Here's how the part is built. I have some questions about the finished solid (model axes, mm). Face numbers are marked on the shaded views. A direction names the side the tool comes from. Coordinates: 2 decimals unless noted, no trailing zeros. Order: outer loops, then holes, each group sorted by start corner. A loop starts at its lowest first (then second) coordinate and runs counter-clockwise, first axis right, second up. Notation, with made-up numbers: M 59,79.25 L 63,79.25 A7 cw 63,92.25 Z; hole C 15,85 d11. An arc over 180 degrees is marked long. One line per question, with ' | ' between items. Start each with the question number.
Autodesk Inventor part; units mm, degrees
ref_plane "YZ Plane" through (0, 0, 0) normal (1, 0, 0) x (0, 1, 0)
ref_plane "XZ Plane" through (0, 0, 0) normal (0, 1, 0) x (-1, 0, 0)
ref_plane "XY Plane" through (0, 0, 0) normal (0, 0, 1) x (1, 0, 0)
sketch "Sketch1" plane through (0, 0, 0) normal (0, 0, 1) x (1, 0, 0)
  line L0 (-4, 16) -> (4, 16)
  line L1 (4, 16) -> (4, -16)
  line L2 (4, -16) -> (-4, -16)
  line L3 (-4, -16) -> (-4, 16)
  point P0 (0, 0)
  dimension "d0" = 8
  dimension "d1" = 32
  dimension "d2" = 4
  dimension "d3" = 16
extrude "Extrusion1" add sketch "Sketch1" along normal blind 3.2
shell "Shell1" thickness 1.5 removed faces 1 at (1.3333, 5.3333, 0)
sketch "Sketch2" plane through (0, 0, 3.2) normal (0, 0, 1) x (1, 0, 0)
  circle A0 centre (0, -12) radius 2.5
  line L0 (4, 16) -> (4, -16)
  line L1 (4, -16) -> (-4, -16)
  dimension "d7" = 5
  dimension "d10" = 4
  dimension "d11" = 4
extrude "Extrusion2" [suppressed]
sketch "Sketch3" plane through (2.5, -14.5, 1.7) normal (0, 0, -1) x (-1, 0, 0)
  circle A0 centre (2.5, 2.5) radius 1.2
  point P0 (2.5, 14.5)
  dimension "d18" = 2.4
extrude "Extrusion3" [suppressed]
pattern_linear "Rectangular Pattern1" [suppressed]
sketch "Sketch4" plane through (2.5, -14.5, 1.7) normal (0, 0, -1) x (-1, 0, 0)
  line L0 (0, 29) -> (0, 0)
  line L1 (0, 0) -> (5, 0)
  circle A0 centre (6.5, 6.5) radius 3.15
  circle A1 centre (6.5, 6.5) radius 2.5
  point P0 (2.5, 14.5)
  dimension "d21" = 6.5
  dimension "d22" = 6.5
  dimension "d25" = 5
  dimension "d26" = 6.3
extrude "Extrusion4" [suppressed]
pattern_linear "Rectangular Pattern2" [suppressed]
equation "\"d0\" = 0.8 * WIDTH"
equation "\"d1\" = 0.8 * LENGTH"
equation "\"d4\" = HEIGHT"
equation "\"d21\" = 0.5 * d23 + 0.5 * d24"
equation "\"d22\" = d21"
equation "\"WIDTH\" = 1"
equation "\"HEIGHT\" = 3.2"
properties part number "2431" material "Steel"
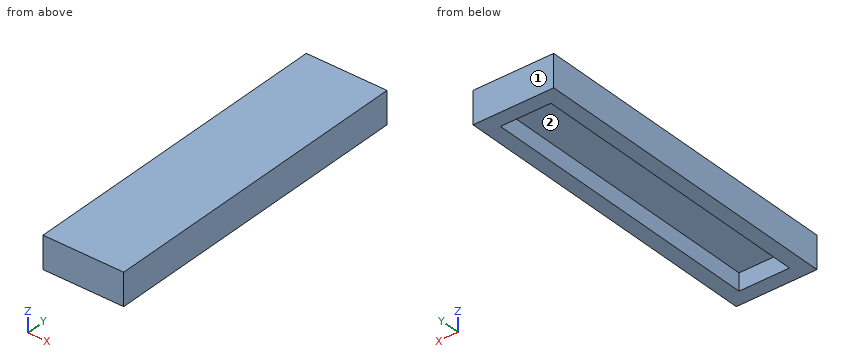
1. Imagine slicing it at A-A (x = 1.75). List the corners of the cut face in (y, z) for me, then the cut area to 3 significant figures.
2. I need wall thicknesses on line 1 (X direction, y = -8, z = 1.2); line 2 (Y direction, x = -1.5, z = 0.45); line 3 (Z direction, x = 2.25, y = -14). Which ranges of each line are inside material? Lowest first, please.
3. Imagine slicing it at B-B (z = 1.2). List the corners of the cut face in (x, y) for me, then the cut area to 3 significant figures.
4. Imagine slicing it at C-C (y = -12). List the corners of the cut face in (x, z) for me.
5. Which directions (+Z, -Z, +X, -X, +Y, -Y) give clear straight access to the entire face, cutting with the end or side of a thin tool? Please do the marked faces 1 and 2.
Entries:
1) outline: M -16,0 L -14.5,0 L -14.5,1.7 L 14.5,1.7 L 14.5,0 L 16,0 L 16,3.2 L -16,3.2 Z | area: 53.1 mm²
2) line 1: -4 to -2.5, 2.5 to 4 | line 2: -16 to -14.5, 14.5 to 16 | line 3: 1.7 to 3.2
3) outline: M -4,-16 L 4,-16 L 4,16 L -4,16 Z; hole M -2.5,-14.5 L 2.5,-14.5 L 2.5,14.5 L -2.5,14.5 Z | area: 111 mm²
4) outline: M -4,0 L -2.5,0 L -2.5,1.7 L 2.5,1.7 L 2.5,0 L 4,0 L 4,3.2 L -4,3.2 Z
5) face 1: +Z, -Z, +X, -X, +Y | face 2: -Z
